Build history of the part. All positions in model axes, mm. Round coordinates to 2 decimals unless told otherwise and drop trailing zeros. Write each loop counter-clockwise with the first axis right and the second up, starting at its lowest first coordinate (ties: lowest second). Pieces come first, ordered by that corner, then holes. Notation, with made-up numbers: (-15, -39.75) -> (19, -39.75) arc R12 ccw to (19, -28.75) -> close; hole circle Ø7 at (21, 61.5). An arc over 180 degrees is marked (long way). Return JSON: item names as keys, results as strings.
from build123d import *

# Parameters (mm, degrees)
SKETCH1_W           = 457.2020066
SKETCH1_H           = 3.175
BOSS_EXTRUDE1_DEPTH = 242.425000036
SKETCH2_W           = 3.175
SKETCH2_H           = 114.3
CUT_EXTRUDE1_DEPTH  = 334.224218774
LPATTERN1_COUNT     = 4
LPATTERN1_PITCH     = 90.807
SKETCH3_W           = 49.658811606
SKETCH3_H           = 3.175
BOSS_EXTRUDE2_DEPTH = 3.175
BOSS_EXTRUDE3_DEPTH = 3.175
SKETCH5_W           = 3.175
SKETCH5_H           = 104.775
CUT_EXTRUDE2_DEPTH  = 3.175


with BuildPart() as part:
    # Sketch1 → Boss-Extrude1 (new body)
    with BuildSketch(Plane.XY):
        Rectangle(SKETCH1_W, SKETCH1_H)
    extrude(amount=BOSS_EXTRUDE1_DEPTH)

    # Sketch2 → Cut-Extrude1 (cut, through all)
    with BuildSketch(Plane(origin=(0, 1.5875, 0), x_dir=(1, 0, 0), z_dir=(0, 1, 0))):
        with Locations((136.2085033, -57.15)):
            Rectangle(SKETCH2_W, SKETCH2_H)
    cut_extrude1 = extrude(amount=-CUT_EXTRUDE1_DEPTH, mode=Mode.SUBTRACT)

    # LPattern1: Cut-Extrude1 ×4
    with Locations(*[(-i * LPATTERN1_PITCH, 0, 0) for i in range(1, LPATTERN1_COUNT)]):
        add(cut_extrude1, mode=Mode.SUBTRACT)

    # Sketch3 → Boss-Extrude2 (add)
    with BuildSketch(Plane(origin=(0, 0, 0), x_dir=(-1, 0, 0), z_dir=(0, 0, -1))):
        with Locations((-91.009597469, 0)):
            Rectangle(SKETCH3_W, SKETCH3_H)
        with Locations((91.030590869, 0)):
            Rectangle(SKETCH3_W, SKETCH3_H)
    extrude(amount=BOSS_EXTRUDE2_DEPTH)

    # Sketch4 → Boss-Extrude3 (add)
    with BuildSketch(Plane.XZ.offset(1.5875)):
        Polygon((-228.6010033, 0), (-266.7010033, 0), (-228.6010033, 50.8), align=None)
    boss_extrude3 = extrude(amount=-BOSS_EXTRUDE3_DEPTH)

    # Mirror1: Boss-Extrude3 across plane
    add(boss_extrude3.mirror(Plane(origin=(0, 0, 0), x_dir=(0, 0, 1), z_dir=(1, 0, 0))))

    # Sketch5 → Cut-Extrude2 (cut)
    with BuildSketch(Plane.XZ.offset(1.5875)):
        with Locations((-227.0135033, 190.037500036)):
            Rectangle(SKETCH5_W, SKETCH5_H)
    cut_extrude2 = extrude(amount=-CUT_EXTRUDE2_DEPTH, mode=Mode.SUBTRACT)

    # Mirror2: Cut-Extrude2 across plane
    add(cut_extrude2.mirror(Plane(origin=(0, 0, 0), x_dir=(0, 0, 1), z_dir=(1, 0, 0))), mode=Mode.SUBTRACT)


solid = part.part
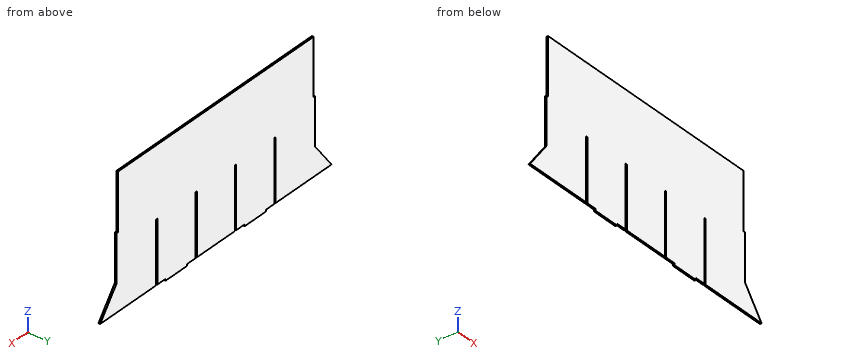
Q1. Saw through at A-A on z = 98. List the corners of the cut face in (x, y) (1 decimal).
Verdict:
{"outline": "(-228.6, -1.6) -> (-137.8, -1.6) -> (-137.8, 1.6) -> (-228.6, 1.6) -> close; (-134.6, -1.6) -> (-47, -1.6) -> (-47, 1.6) -> (-134.6, 1.6) -> close; (-43.8, -1.6) -> (43.8, -1.6) -> (43.8, 1.6) -> (-43.8, 1.6) -> close; (47, -1.6) -> (134.6, -1.6) -> (134.6, 1.6) -> (47, 1.6) -> close; (137.8, -1.6) -> (228.6, -1.6) -> (228.6, 1.6) -> (137.8, 1.6) -> close"}
Q2. Saw through at C-C on z = 152.5. List the corners of the cut face in (x, y).
Verdict:
{"outline": "(-225.43, -1.59) -> (225.43, -1.59) -> (225.43, 1.59) -> (-225.43, 1.59) -> close"}
Q3. Wall check: L1, parallel to X at y = -0.35, z = 62 (3 decimals); L2, parallel to X at y = -0.2, z = 13.5 (3 decimals); L3, parallel to Z at x = -56, y = 0.35 (3 decimals). Give the ranges that are in metal, low to high.
Verdict:
{"L1": "x = -228.601 to -137.8, -134.625 to -46.993, -43.818 to 43.814, 46.989 to 134.621, 137.796 to 228.601", "L2": "x = -256.576 to -137.8, -134.625 to -46.993, -43.818 to 43.814, 46.989 to 134.621, 137.796 to 256.576", "L3": "z = 0 to 242.425"}
Q4. Pin check, flat tips, straight feed: pin 1 Ø1.6 at (y, z) = (0, 38) entering from -X; pin 2 Ø1 at (y, z) = (0, 92) entering from -X; pin 3 Ø1 at (x, y) = (157, -1) entering from -Z. Stop position of each tip, or through.
Verdict:
{"pin 1": "stops at x = -238.8", "pin 2": "stops at x = -228.6", "pin 3": "stops at z = 0"}
